```python
from build123d import *

# Parameters (mm, degrees)
F0_W     = 20
F0_H     = 10
F1_DEPTH = 4
F2_R     = 5


with BuildPart() as f1:
    # F0 (on Top) → F1 (new body)
    with BuildSketch(Plane.XY):
        Polygon((5, -15), (5, 15), (-5, 15), (-5, 5), (-5, -15), align=None)
        with Locations((-15, 10)):
            Rectangle(F0_W, F0_H)
    extrude(amount=F1_DEPTH)

    # F2
    f2_edges = [f1.edges().sort_by_distance(p)[0] for p in [
        (5, 15, 2),
    ]]
    fillet(f2_edges, radius=F2_R)


solid = f1.part
```
Read the model definition and answer for the solid it produces. Units are mm, in the model's axes. A direction names the side the tool comes from. Coordinates: 2 decimals unless noted, no trailing zeros. Write each loop counter-clockwise with the first axis right and the second up, starting at its lowest first coordinate (ties: lowest second). Pieces come first, ordered by that corner, then holes. Notation, with made-up numbers: (28, -15.75) -> (63, -15.75) arc R31 cw to (63, 21.25) -> close; hole circle Ø2 at (89.25, 11.5). An arc over 180 degrees is marked (long way). Answer as a JSON object with one key per item and string values.
Q1. Flat-ended cylindrical pins translate along their axes: pin 1 Ø1 at (y, z) = (-1.5, 1.5) entering from -X; pin 2 Ø1.2 at (x, z) = (-17.5, 2.5) entering from -Y. Find the tip coordinate at first contact, or state that the pin passes through.
The answers:
{"pin 1": "stops at x = -5", "pin 2": "stops at y = 5"}
Q2. A tool of negligible diameter and unlimited length cuts with its end or side. For faces 1 (the flat face through (-15, 5, 2)), 2 (the flat face through (-4, 4, 0)), from which of +Z, -Z, +X, -X, +Y, -Y can it reach the whole face along a straight path? Write none if from no direction.
The answers:
{"face 1": "+Z, -Z, -X, -Y", "face 2": "-Z, +X, -X, +Y, -Y"}
Q3. The part is cut by section C-C on y = 0.25. Give the vertices of the cut face in (x, z), then the cut area to 3 significant figures.
The answers:
{"outline": "(-5, 0) -> (5, 0) -> (5, 4) -> (-5, 4) -> close", "area": "40.0 mm2"}
Q4. The part is cut by section A-A on z = 2.9. Give the vertices of the cut face in (x, y).
The answers:
{"outline": "(-25, 5) -> (-5, 5) -> (-5, -15) -> (5, -15) -> (5, 10) arc R5 ccw to (0, 15) -> (-25, 15) -> close"}
Q5. The part is cut by section B-B on x = -21.75. Give the vertices of the cut face in (y, z).
The answers:
{"outline": "(5, 0) -> (15, 0) -> (15, 4) -> (5, 4) -> close"}
Q6. Consider line 1 (Y direction, x = -22.25, z = 1.7); line 2 (X direction, y = -13.5, z = 0.7); line 3 (X direction, y = 11.5, z = 0.4). Determine where each line is inside the solid, lowest interval first. Write a range as [from, to].
The answers:
{"line 1": "y = [5, 15]", "line 2": "x = [-5, 5]", "line 3": "x = [-25, 4.77]"}
